Autodesk Inventor part; units mm, degrees
ref_plane "YZ Plane" through (0, 0, 0) normal (1, 0, 0) x (0, 1, 0)
ref_plane "XZ Plane" through (0, 0, 0) normal (0, 1, 0) x (-1, 0, 0)
ref_plane "XY Plane" through (0, 0, 0) normal (0, 0, 1) x (1, 0, 0)
sketch "Sketch2" plane through (0, 0, 0) normal (0, 1, 0) x (-1, 0, 0)
  line L0 (0, 0) -> (0, -65)
  line L1 (0, 0) -> (22, 0)
  line L2 (22, 0) -> (22, -40.3)
  line L3 (22, -40.3) -> (0, -65)
  dimension "d4" = 65
  dimension "d5" = 22
  dimension "d6" = 40.3
revolve "Revolution1" add sketch "Sketch2" angle 360 about axis through (0, 0, 0) along (-1, 0, 0)
sketch "Sketch3" plane through (-22, 0, 0) normal (-1, 0, 0) x (0, 0, 1)
  circle A0 centre (0, 0) radius 40.3
  line L0 (0, 40.3) -> (0, 64.3)
  line L1 (0, 64.3) -> (-7.5, 64.3)
  line L2 (-7.5, 64.3) -> (-7.5, 39.596)
  line L3 (0, 64.3) -> (7.4, 64.3)
  line L4 (7.4, 64.3) -> (7.5, 39.596)
  arc A1 (7.5, 39.596) -> (-7.5, 39.596) centre (0, 0) ccw
  dimension "d11" = 24
  dimension "d12" = 7.5
  dimension "d13" = 7.4
extrude "Extrusion1" cut sketch "Sketch3" against normal blind 10 contours A0 L0 L3 L4 | L2 L1 L0 A0
properties part number "Handle Gearbox" material "PC/ABS Plastic"
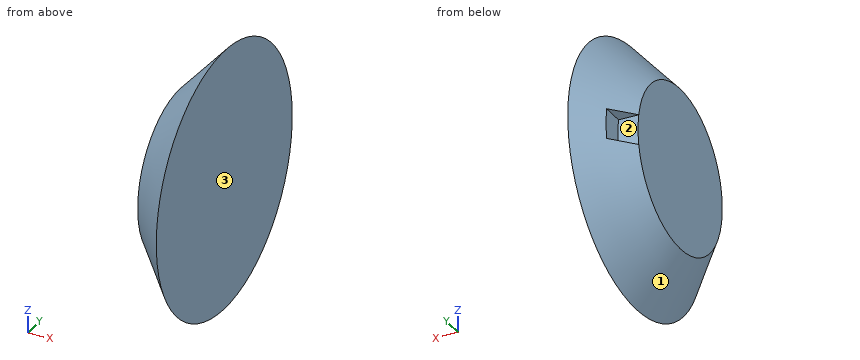
Build history of the part. All positions in model axes, mm. Face numbers are marked on the shaded views. Round coordinates to 2 decimals unless told otherwise and drop trailing zeros. Write each loop counter-clockwise with the first axis right and the second up, starting at its lowest first coordinate (ties: lowest second). Pieces come first, ordered by that corner, then holes. Notation, with made-up numbers: M -40,6 L -27,6 A8 ccw -27,18 Z; hole C 40,26 d6. An arc over 180 degrees is marked long. Answer in a Markdown table with one row per item.
1. Mould opens along Z. For the marked faces 1, 2 and 3 say: +Z half, -Z half, draft (parallel to the pull), parting line (faces both ways), or undercut.
Geometry check:
| item | result |
|---|---|
| face 1 | parting line |
| face 2 | undercut |
| face 3 | draft |
2. Saw through at B-B (y = 0). List the corners of the cut face in (x, z), and give its area (3 significant figures).
Geometry check:
| item | result |
|---|---|
| outline | M -22,-40.3 L 0,-65 L 0,65 L -22,40.3 Z |
| area | 2,320 mm2 |
3. Saw through at D-D (x = -6.75). List the corners of the cut face in (y, z), and give its area (3 significant figures).
Geometry check:
| item | result |
|---|---|
| outline | C 0,0 d114.84 |
| area | 10,400 mm2 |
4. Flat gauge pins, fed straight in: P1, Ø12, axis at x = -8, y = -46.5, coming from the -Z side; P2, Ø1, axis at y = 6, z = 47, coming from the -X side; P3, Ø6, axis at x = -4.5, y = 31, coming from the +Z side. Where does each tip first touch, or does it go through?
Geometry check:
| item | result |
|---|---|
| P1 | z = -43.98 |
| P2 | x = -16.14 |
| P3 | z = 55.55 |
5. Saw through at A-A (z = 0). List the corners of the cut face in (x, y), and give its area (3 significant figures).
Geometry check:
| item | result |
|---|---|
| outline | M -22,-40.3 L 0,-65 L 0,65 L -12,51.53 L -12,40.3 L -22,40.3 Z |
| area | 2,260 mm2 |
6. Saw through at C-C (x = -17.75). List the corners of the cut face in (y, z).
Geometry check:
| item | result |
|---|---|
| outline | M 39.6,-7.5 A40.3 ccw 39.6,7.5 L 44.45,7.48 A45.07 ccw long 44.44,-7.5 Z |
7. Probe L1, parallel to Z at x = -13.5, y = -14; L2, parallel to Z at x = -19.25, y = -29; L3, parallel to Y at x = -1.25, z = -52.5. List the from-to ranges inside material, lowest first. Write a range as [from, to].
Geometry check:
| item | result |
|---|---|
| L1 | [-47.84, 47.84] |
| L2 | [-32.27, 32.27] |
| L3 | [-35.89, 35.89] |
